Verification items for the finished model (mm, model axes). Coordinates: 2 decimals unless noted, no trailing zeros. Order: outer loops, then holes, each group sorted by start corner. A loop starts at its lowest first (then second) coordinate and runs counter-clockwise, first axis right, second up. Notation, with made-up numbers: M 13,-32.5 L 64,-32.5 A14 ccw 64,-27.5 Z; hole C 74.5,-8 d4. An arc over 180 degrees is marked long. Answer as a JSON object with one key per item and string values. Group by question number.
(1) Material ranges on line 1 (X direction, y = -26, z = 2.35); line 2 (Y direction, x = -55, z = 0.1); line 3 (Y direction, x = -38, z = 2.9), recorded low to high.
(2) Cross-section at B-B (y = 25). Enter the section's corners in (x, z), plus the area to 3 significant figures.
(3) Cross-section at C-C (z = 1.25). Count the separate pieces of the cut face and the enclosed holes in it, plus the area to 3 significant figures.
(4) Mould release check, pull along X, two halves, no side actions. Record for faces 1 (the face through (-1, -1, 3)), 2 (the face through (-74.5, 24.84, 1.48)), 3 (the face through (4.5, 25.16, 1.48)): released by +X, released by -X, zero draft, split by the parting line, or undercut.
(5) Cross-section at A-A (x = -43.5). Enter the section's corners in (y, z).
(6) Gauge pin test, flat end, axial feed: pin 1 Ø1.5 at (x, z) = (68.5, 2.5) entering from -Y. Record the tip position at first contact, or that the pin passes through.
from build123d import *

# Parameters (mm, degrees)
SKETCH1_W           = 3
SKETCH1_H           = 20
BOSS_EXTRUDE1_DEPTH = 3


with BuildPart() as part:
    # Sketch1 → Boss-Extrude1 (new body)
    with BuildSketch(Plane.XY):
        Polygon((-100, -50), (-60, -50), (-60, -53), (-40, -53), (-40, -50), (-10, -50), (-10, -53), (10, -53), (10, -50), (40, -50), (40, -53), (60, -53), (60, -50), (100, -50), (100, 50), (-100, 50), align=None)
        with BuildLine():
            Line((-67, -25), (-3, -25))
            ThreePointArc((-3, -25), (-0.878679656, -24.121320344), (0, -22))
            Line((0, -22), (0, -8))
            ThreePointArc((0, -8), (-0.878679656, -5.878679656), (-3, -5))
            Line((-3, -5), (-67, -5))
            ThreePointArc((-67, -5), (-69.121320344, -5.878679656), (-70, -8))
            Line((-70, -8), (-70, -22))
            ThreePointArc((-70, -22), (-69.121320344, -24.121320344), (-67, -25))
        make_face(mode=Mode.SUBTRACT)
        with Locations((-97, 25)):
            Rectangle(SKETCH1_W, SKETCH1_H, mode=Mode.SUBTRACT)
        with Locations((-97, 0)):
            Rectangle(SKETCH1_W, SKETCH1_H, mode=Mode.SUBTRACT)
        with Locations((-97, -25)):
            Rectangle(SKETCH1_W, SKETCH1_H, mode=Mode.SUBTRACT)
        with Locations((97, 25.11339046)):
            Rectangle(SKETCH1_W, SKETCH1_H, mode=Mode.SUBTRACT)
        with Locations((97, 0)):
            Rectangle(SKETCH1_W, SKETCH1_H, mode=Mode.SUBTRACT)
        with Locations((97, -25)):
            Rectangle(SKETCH1_W, SKETCH1_H, mode=Mode.SUBTRACT)
        with BuildLine():
            Line((17.066389082, 37.5), (42.066389082, 37.5))
            ThreePointArc((42.066389082, 37.5), (44.452998622, 35.11339046), (42.066389082, 32.72678092))
            Line((42.066389082, 32.72678092), (17.066389082, 32.72678092))
            ThreePointArc((17.066389082, 32.72678092), (14.679779542, 35.11339046), (17.066389082, 37.5))
        make_face(mode=Mode.SUBTRACT)
        with BuildLine():
            Line((17.066389082, 20.00057963), (42.066389082, 20.00057963))
            ThreePointArc((42.066389082, 20.00057963), (44.566389082, 17.50057963), (42.066389082, 15.00057963))
            Line((42.066389082, 15.00057963), (17.066389082, 15.00057963))
            ThreePointArc((17.066389082, 15.00057963), (14.566389082, 17.50057963), (17.066389082, 20.00057963))
        make_face(mode=Mode.SUBTRACT)
        with BuildLine():
            Line((17.066389082, 3.766162691), (42.066389082, 3.766162691))
            ThreePointArc((42.066389082, 3.766162691), (44.566389082, 1.266162691), (42.066389082, -1.233837309))
            Line((42.066389082, -1.233837309), (17.066389082, -1.233837309))
            ThreePointArc((17.066389082, -1.233837309), (14.566389082, 1.266162691), (17.066389082, 3.766162691))
        make_face(mode=Mode.SUBTRACT)
        with BuildLine():
            Line((16.882588886, -32.5), (41.882588886, -32.5))
            ThreePointArc((41.882588886, -32.5), (44.382588886, -35), (41.882588886, -37.5))
            Line((41.882588886, -37.5), (16.882588886, -37.5))
            ThreePointArc((16.882588886, -37.5), (14.382588886, -35), (16.882588886, -32.5))
        make_face(mode=Mode.SUBTRACT)
        with BuildLine():
            Line((17.066389082, -12.5), (42.066389082, -12.5))
            ThreePointArc((42.066389082, -12.5), (44.566389082, -15), (42.066389082, -17.5))
            Line((42.066389082, -17.5), (17.066389082, -17.5))
            ThreePointArc((17.066389082, -17.5), (14.566389082, -15), (17.066389082, -12.5))
        make_face(mode=Mode.SUBTRACT)
        with BuildLine():
            Line((-67, 32.5), (-3, 32.5))
            ThreePointArc((-3, 32.5), (4.5, 25), (-3, 17.5))
            Line((-3, 17.5), (-67, 17.5))
            ThreePointArc((-67, 17.5), (-74.5, 25), (-67, 32.5))
        make_face(mode=Mode.SUBTRACT)
        with BuildLine():
            Line((-67, -32.5), (-3, -32.5))
            ThreePointArc((-3, -32.5), (-0.5, -35), (-3, -37.5))
            Line((-3, -37.5), (-67, -37.5))
            ThreePointArc((-67, -37.5), (-69.5, -35), (-67, -32.5))
        make_face(mode=Mode.SUBTRACT)
    extrude(amount=BOSS_EXTRUDE1_DEPTH)


solid = part.part
Taken from the geometry:
{
 "1": {"line 1": "x = -100 to -98.5, -95.5 to 95.5, 98.5 to 100", "line 2": "y = -53 to -37.5, -32.5 to -25, -5 to 17.5, 32.5 to 50", "line 3": "y = -50 to -37.5, -32.5 to -25, -5 to 17.5, 32.5 to 50"},
 "2": {"outline": "M -100,0 L -98.5,0 L -98.5,3 L -100,3 Z; M -95.5,0 L -74.5,0 L -74.5,3 L -95.5,3 Z; M 4.5,0 L 95.5,0 L 95.5,3 L 4.5,3 Z; M 98.5,0 L 100,0 L 100,3 L 98.5,3 Z", "area": "345 mm²"},
 "3": {"separate pieces": "1", "enclosed holes": "14", "area": "16,200 mm²"},
 "4": {"face 1": "zero draft", "face 2": "undercut", "face 3": "undercut"},
 "5": {"outline": "M -53,0 L -37.5,0 L -37.5,3 L -53,3 Z; M -32.5,0 L -25,0 L -25,3 L -32.5,3 Z; M -5,0 L 17.5,0 L 17.5,3 L -5,3 Z; M 32.5,0 L 50,0 L 50,3 L 32.5,3 Z"},
 "6": {"pin 1": "stops at y = -50"}
}
